The drawing under review shows one solid part. Ordinate dimensions are in mm from its lowest x, y, z. A direction names the side the tool comes from. Round coordinates to 2 decimals unless told otherwise and drop trailing zeros. Write each loop counter-clockwise with the first axis right and the second up, starting at its lowest first coordinate (ties: lowest second). Pieces come first, ordered by that corner, then holes.
Item 1: Add section A-A (z = 22.5). Give the boundary of the cut face in (x, y).
Item 2: Clearance check with flat-ended pins moving along their axes: pin 1 Ø1 at (y, z) = (8, 54) entering from +X; pin 2 Ø5 at (y, z) = (11, 62) entering from -X; pin 3 Ø1.5 at (x, z) = (31, 35.5) entering from +Y. State where each tip first meets the part, or that it passes through.
Item 3: Add section B-B (x = 30). Give the boundary of the cut face in (y, z), plus the area to 3 significant figures.
Item 4: To check wall thickness, follow L1, parallel to Z at x = 30, y = 16.75; L2, parallel to X at y = 13, z = 35; L3, parallel to X at y = 15.25, z = 35. State the ranges of each line that lie inside material, in increasing order.
Item 5: Machinability: for the marked faces 1, 2 and 3, which of the approach directions +Z, -Z, +X, -X, +Y, -Y give a long, thin tool a straight path to every point of the face, cutting with its end or side? Answer none if there is none.
Item 6: Add section D-D (y = 8.75). Give the boundary of the cut face in (x, z), plus the area to 3 significant figures.
Item 7: Add section C-C (y = 13.25). Give the boundary of the cut face in (x, z), plus the area to 3 significant figures.
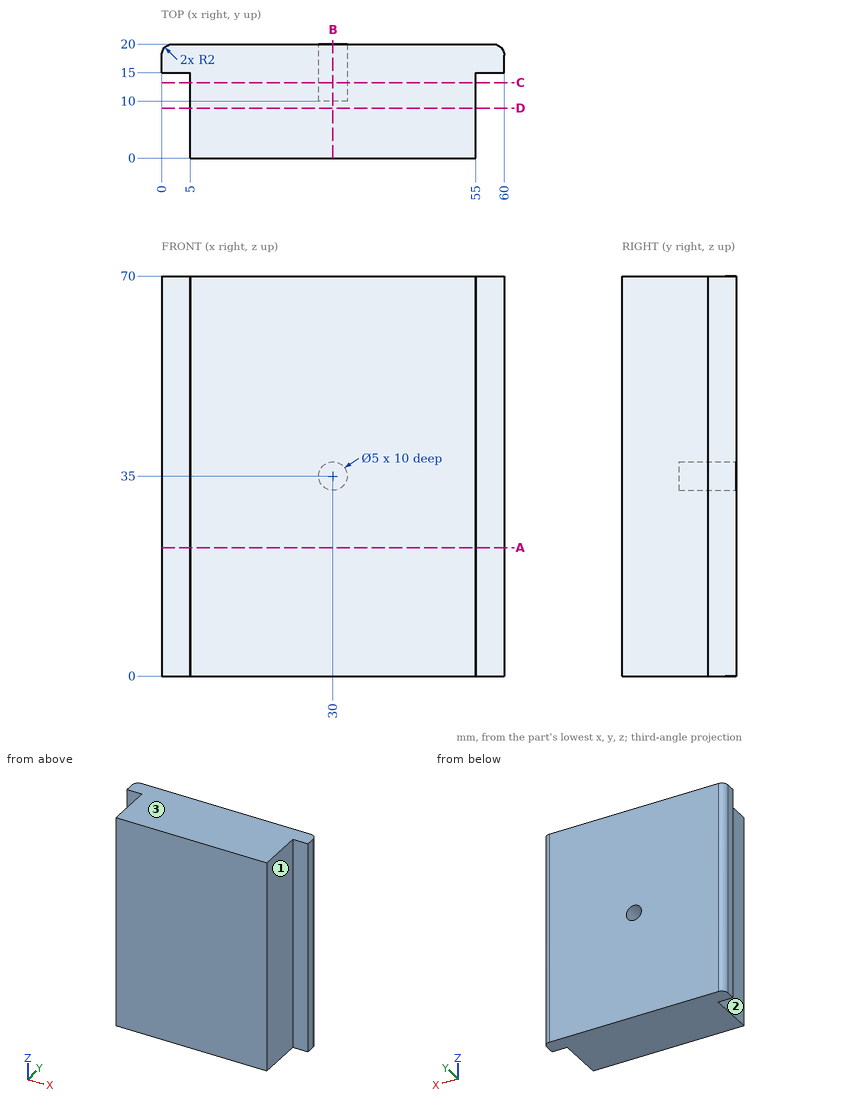
Numbers:
1. outline: (0, 15) - (5, 15) - (5, 0) - (55, 0) - (55, 15) - (60, 15) - (60, 18) arc R2 ccw to (58, 20) - (2, 20) arc R2 ccw to (0, 18) - close
2. pin 1: stops at x = 55
2. pin 2: stops at x = 5
2. pin 3: stops at y = 10
3. outline: (0, 0) - (20, 0) - (20, 32.5) - (10, 32.5) - (10, 37.5) - (20, 37.5) - (20, 70) - (0, 70) - close
3. area: 1,350 mm2
4. L1: z = 0 to 32.5, 37.5 to 70
4. L2: x = 5 to 27.5, 32.5 to 55
4. L3: x = 0 to 27.5, 32.5 to 60
5. face 1: +Z, -Z, +X, -Y
5. face 2: +Z, -Z, -X, -Y
5. face 3: +Z, +X, -X, +Y, -Y
6. outline: (5, 0) - (55, 0) - (55, 70) - (5, 70) - close
6. area: 3,500 mm2
7. outline: (5, 0) - (55, 0) - (55, 70) - (5, 70) - close; hole circle Ø5 at (30, 35)
7. area: 3,480 mm2
